The model under review builds one solid part; all positions refer to its coordinate system, in mm. Coordinates: 2 decimals unless noted, no trailing zeros. Loops run counter-clockwise (first coordinate to the right, second up) from the corner with the lowest first, then second, coordinate; pieces in that order, holes last. Notation, with made-up numbers: M 62,51 L 108,51 A14 cw 108,67 Z; hole C 12.5,13 d6. An arc over 180 degrees is marked long. One line per item, written item: value.
```python
from build123d import *

# Parameters (mm, degrees)
SKETCH1_R           = 2.125
BOSS_EXTRUDE1_DEPTH = 2


with BuildPart() as part:
    # Sketch1 → Boss-Extrude1 (new body)
    with BuildSketch(Plane(origin=(0, 0, 0), x_dir=(1, 0, 0), z_dir=(0, 1, 0))):
        with BuildLine():
            Line((-37.655823606, 28.125414637), (-49.673639651, 37.101610798))
            ThreePointArc((-49.673639651, 37.101610798), (-59.88740123, 16.046780796), (-61.569439235, -7.294117647))
            Line((-61.569439235, -7.294117647), (-46.673607162, -5.529411765))
            ThreePointArc((-46.673607162, -5.529411765), (-45.398513836, 12.16449512), (-37.655823606, 28.125414637))
        make_face()
        with Locations((-44.167295593, 25.5)):
            Circle(SKETCH1_R, mode=Mode.SUBTRACT)
        with Locations((-51.095498823, 29.5)):
            Circle(SKETCH1_R, mode=Mode.SUBTRACT)
        with Locations((-59, 0)):
            Circle(SKETCH1_R, mode=Mode.SUBTRACT)
        with Locations((-51, 0)):
            Circle(SKETCH1_R, mode=Mode.SUBTRACT)
    extrude(amount=BOSS_EXTRUDE1_DEPTH)


solid = part.part
```
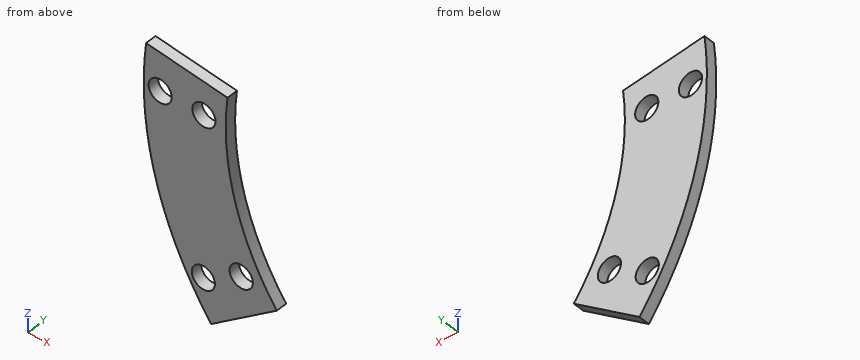
(1) Add section D-D on z = -25.5. State the section outline as (x, y) points.
Checks:
outline: M -56.51,0 L -46.29,0 L -46.29,2 L -56.51,2 Z; M -42.04,0 L -39.48,0 L -39.48,2 L -42.04,2 Z
(2) Add section A-A on z = 0. State the section outline as (x, y) points (3 decimals), then the cut area to 3 significant figures.
Checks:
outline: M -62,0 L -61.125,0 L -61.125,2 L -62,2 Z; M -56.875,0 L -53.125,0 L -53.125,2 L -56.875,2 Z; M -48.875,0 L -47,0 L -47,2 L -48.875,2 Z
area: 13.0 mm^2
(3) Add section B-B on y = 0.4. State how many separate pieces and enclosed holes the cut face has, then the cut area to 3 significant figures.
Checks:
separate pieces: 1
enclosed holes: 4
area: 564 mm^2
(4) Add section C-C on x = -44.25. State the section outline as (y, z) points, then the cut area to 3 significant figures.
Checks:
outline: M 0,-33.05 L 2,-33.05 L 2,-27.62 L 0,-27.62 Z; M 0,-23.38 L 2,-23.38 L 2,-15.84 L 0,-15.84 Z
area: 25.9 mm^2
(5) To check wall thickness, follow L1, parallel to X at y = 1.1, z = 0 (3 decimals); L2, parallel to Z at x = -49.25, y = 1.2; L3, parallel to Z at x = -51, y = 1.3 (3 decimals). State the ranges of each line that lie inside material, in increasing order. Write a range as [from, to].
Checks:
L1: [-62, -61.125], [-56.875, -53.125], [-48.875, -47]
L2: [-36.79, -30.55], [-28.45, -1.21], [1.21, 5.83]
L3: [-35.256, -31.623], [-27.377, -2.125], [2.125, 6.042]
(6) Insertion check: pin 1 Ø1 at (x, y) = (-48.5, 2) entering from +Z (3 decimals); pin 2 Ø5.5 at (x, z) = (-44.17, -25.5) entering from +Y. Each pin has a flat end and moves straight along its axis. Give the tip position at first contact, or say it passes through.
Checks:
pin 1: z = 5.805
pin 2: y = 2
